Geometry check sheet. Reference: the model listing, model coordinates, mm. A direction names the side the tool comes from. Coordinates: 2 decimals unless noted, no trailing zeros. Write each loop counter-clockwise with the first axis right and the second up, starting at its lowest first coordinate (ties: lowest second). Pieces come first, ordered by that corner, then holes.
Autodesk Inventor part; units mm, degrees
ref_plane "YZ Plane" through (0, 0, 0) normal (1, 0, 0) x (0, 1, 0)
ref_plane "XZ Plane" through (0, 0, 0) normal (0, 1, 0) x (-1, 0, 0)
ref_plane "XY Plane" through (0, 0, 0) normal (0, 0, 1) x (1, 0, 0)
sketch "Sketch1" plane through (0, 0, 0) normal (0, 0, 1) x (1, 0, 0)
  circle A0 centre (0, 0) radius 5.5
  circle A1 centre (0, 0) radius 22.5
  dimension "d0" = 11
  dimension "d1" = 45
extrude "Extrusion1" add sketch "Sketch1" along normal blind 120
sketch "Sketch2" plane through (0, 0, 120) normal (0, 0, 1) x (1, 0, 0)
  circle A0 centre (0, 0) radius 25
  circle A1 centre (0, 0) radius 5.5
  dimension "d4" = 50
  dimension "d5" = 11
extrude "Extrusion2" add sketch "Sketch2" against normal blind 7
sketch "Sketch3" plane through (0, 0, 0) normal (0, 0, -1) x (-1, 0, 0)
  circle A0 centre (0, 0) radius 5.5
  circle A1 centre (0, 0) radius 25
  dimension "d8" = 11
  dimension "d9" = 50
extrude "Extrusion3" add sketch "Sketch3" against normal blind 7
sketch "Sketch4" plane through (0, 0, 0) normal (0, 0, -1) x (-1, 0, 0)
  circle A0 centre (0, 0) radius 5.5
  circle A1 centre (0, 0) radius 10
  dimension "d12" = 20
extrude "Extrusion4" add sketch "Sketch4" along normal blind 5
sketch "Sketch5" plane through (0, 0, 120) normal (0, 0, 1) x (1, 0, 0)
  circle A0 centre (0, 0) radius 5.5
  circle A1 centre (0, 0) radius 10
  dimension "d15" = 20
extrude "Extrusion5" add sketch "Sketch5" along normal blind 15
properties part number "Ydre"
1. Sectioned sample at C-C, the plane x = -12.5. Record the boundary of the cut face in (y, z).
Computed values:
outline: (-21.65, 0) - (21.65, 0) - (21.65, 7) - (18.71, 7) - (18.71, 113) - (21.65, 113) - (21.65, 120) - (-21.65, 120) - (-21.65, 113) - (-18.71, 113) - (-18.71, 7) - (-21.65, 7) - close
2. Access from +Z, -Z, +X, -X, +Y, -Y to the whole of each face (thin tool, end or side, straight path). Record for faces 5 (the flat face through (22.34, 3.82, 7)), 6 (the flat face through (0, -11, 120)), 7 (the cylindrical face through (2.17, 9.76, -2.46)).
Computed values:
face 5: none
face 6: +Z
face 7: -Z
3. Gauge pin test, flat ends, axial feed: pin 1 Ø3 at (x, z) = (-9.5, 17) entering from +Y; pin 2 Ø5 at (x, y) = (15, -17) entering from -Z; pin 3 Ø4 at (y, z) = (-6, 37) entering from +X. Record the tip position at first contact, or that the pin passes through.
Computed values:
pin 1: stops at y = 21.03
pin 2: stops at z = 0
pin 3: stops at x = 22.14
4. Thickness scan on line 1 along Y through (x, z) = (0, 48); line 2 along Y through (x, z) = (0, 128); line 3 along Z through (x, y) = (-20, 5). Record the ranges inside material, lowest first.
Computed values:
line 1: y = -22.5 to -5.5, 5.5 to 22.5
line 2: y = -10 to -5.5, 5.5 to 10
line 3: z = 0 to 120
5. Draft check along Z on faces 1 (the cylindrical face through (10.382, 19.961, 59.258)), 2 (the flat face through (0, -11, 0)), 3 (the cylindrical face through (-2.17, 9.76, 127.4)), 4 (the flat face through (-22.34, 3.82, 113)). Enter one of: released by +Z, released by -Z, zero draft, split by the parting line, or undercut.
Computed values:
face 1: undercut
face 2: released by -Z
face 3: zero draft
face 4: undercut
6. Sectioned sample at D-D, the plane y = -8. Record the boundary of the cut face in (x, z), and give its area (3 significant figures).
Computed values:
outline: (-23.69, 0) - (-6, 0) - (-6, -5) - (6, -5) - (6, 0) - (23.69, 0) - (23.69, 7) - (21.03, 7) - (21.03, 113) - (23.69, 113) - (23.69, 120) - (6, 120) - (6, 135) - (-6, 135) - (-6, 120) - (-23.69, 120) - (-23.69, 113) - (-21.03, 113) - (-21.03, 7) - (-23.69, 7) - close
area: 5,360 mm2
7. Sectioned sample at A-A, the plane x = 0. Record the boundary of the cut face in (y, z).
Computed values:
outline: (-25, 0) - (-10, 0) - (-10, -5) - (-5.5, -5) - (-5.5, 135) - (-10, 135) - (-10, 120) - (-25, 120) - (-25, 113) - (-22.5, 113) - (-22.5, 7) - (-25, 7) - close; (5.5, -5) - (10, -5) - (10, 0) - (25, 0) - (25, 7) - (22.5, 7) - (22.5, 113) - (25, 113) - (25, 120) - (10, 120) - (10, 135) - (5.5, 135) - close
